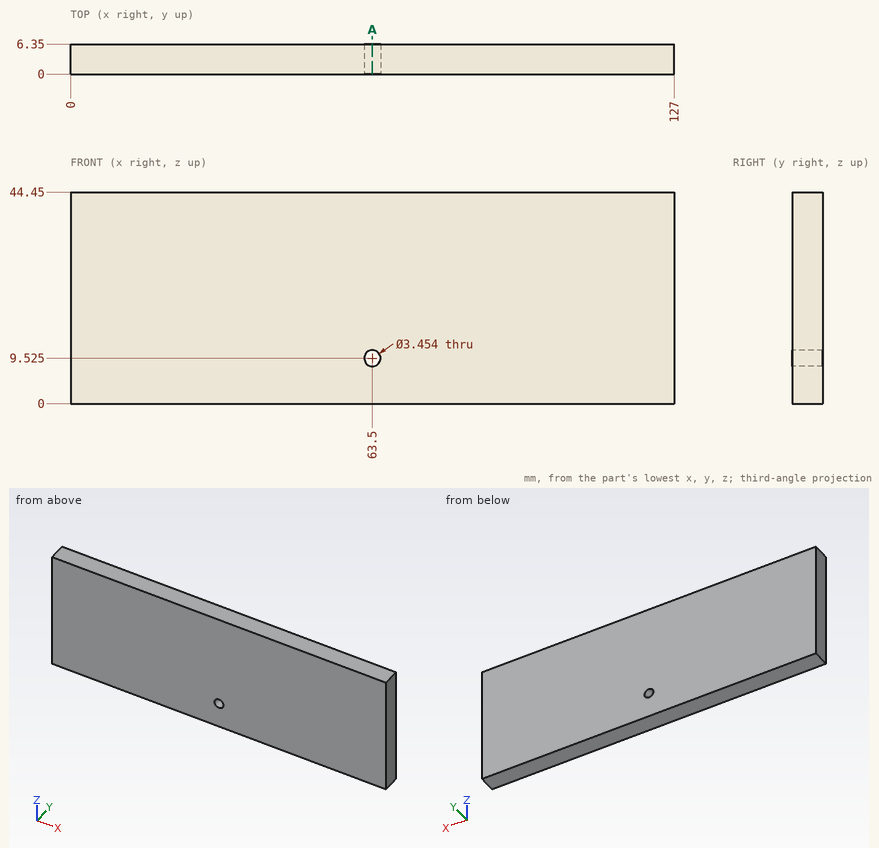
Geometry check sheet. Reference: drawing and pictorial views, mm from the part's lowest x, y, z. Coordinates: 2 decimals unless noted, no trailing zeros. Loops run counter-clockwise (first coordinate to the right, second up) from the corner with the lowest first, then second, coordinate; pieces in that order, holes last. Notation, with made-up numbers: (19.25, 66) -> (32.25, 66) arc R12 ccw to (32.25, 84) -> close; hole circle Ø4 at (4, -13.5). An arc over 180 degrees is marked (long way). Write item = value, one per line. Start each with the question number.
1. Depth check by flat-ended pin: P1, Ø8, axis at x = 72.5, z = 20, coming from the -Y side; P2, Ø3, axis at x = 63.5, z = 9.525, coming from the -Y side. Enter the tip coordinate at first touch or a pass-through.
2. Section check A-A on x = 63.5. Record the cut outline in (y, z), then the cut area to 3 significant figures.
3. Material ranges on line 1 (X direction, y = 5, z = 11), recorded low to high.
Responses:
q1.P1 = 0
q1.P2 = through
q2.outline = (0, 0) -> (6.35, 0) -> (6.35, 7.8) -> (0, 7.8) -> close; (0, 11.25) -> (6.35, 11.25) -> (6.35, 44.45) -> (0, 44.45) -> close
q2.area = 260 mm2
q3.line_1 = 0 to 62.6, 64.4 to 127
